Check sheet for the modelled part. Datum: model origin and axes. Units: mm. A direction names the side the tool comes from. Coordinates: 2 decimals unless noted, no trailing zeros. Loops run counter-clockwise (first coordinate to the right, second up) from the corner with the lowest first, then second, coordinate; pieces in that order, holes last.
from build123d import *

# Parameters (mm, degrees)
BOSS_EXTRUDE1_DEPTH = 10


# Read off the part's stored shape, not the designer's step: Imported1
with BuildPart() as part:
    # Sketch3 → Boss-Extrude1 (new body)
    with BuildSketch(Plane(origin=(14.999999665, 0, 0), x_dir=(0, 0, -1), z_dir=(1, 0, 0))):
        with BuildLine():
            Line((29.553098604, 349.581092596), (28.873996809, 356.511801481))
            ThreePointArc((28.873996809, 356.511801481), (26.617852211, 359.926750423), (22.636385635, 360.875427723))
            Line((22.636385635, 360.875427723), (-5.304185674, 354.369103909))
            Line((-5.304185674, 354.369103909), (-10.304185562, 354.369103909))
            Line((-10.304185562, 354.369103909), (-10.304185562, 214.764729142))
            Line((-10.304185562, 214.764729142), (43.492022902, 215.872973204))
            ThreePointArc((43.492022902, 215.872973204), (47.063645136, 218.78911025), (48.163164407, 223.266988993))
            Line((48.163164407, 223.266988993), (46.73166573, 228.318288922))
            Line((46.73166573, 228.318288922), (44.741906226, 228.116184473))
            Line((44.741906226, 228.116184473), (45.146130025, 224.136650562))
            Line((45.146130025, 224.136650562), (43.445847929, 219.970226288))
            Line((43.445847929, 219.970226288), (38.855373859, 219.58476305))
            Line((38.855373859, 219.58476305), (38.622945547, 221.872985363))
            Line((38.622945547, 221.872985363), (5.372944754, 221.872985363))
            Line((5.372944754, 221.872985363), (5.372944288, 349.872976542))
            Line((5.372944288, 349.872976542), (20.103313029, 353.819966316))
            Line((20.103313029, 353.819966316), (19.735585898, 356.090396643))
            Line((19.735585898, 356.090396643), (24.27472733, 356.836169958))
            Line((24.27472733, 356.836169958), (26.93930082, 353.209882975))
            Line((26.93930082, 353.209882975), (27.578826994, 349.261313677))
            Line((27.578826994, 349.261313677), (29.553098604, 349.581092596))
        make_face()
        Polygon((-5.304185562, 221.872985363), (0.372943822, 221.872985363), (0.372943822, 348.53323067), (-5.304185562, 347.01204868), align=None, mode=Mode.SUBTRACT)
    extrude(amount=BOSS_EXTRUDE1_DEPTH)


solid = part.part
(1) Section check D-D, the plane y = 226. Enter the section's corners in (x, z), plus the area to 3 significant figures.
(2) Scan lines: line 1 along Z through (x, y) = (24, 237); line 2 along Y through (x, z) = (19.75, -26.5); line 3 along Y through (x, z) = (20.5, -10.5). Record each from-to range of solid material in increasing order.
(3) Gauge pin test, flat ends, axial feed: P1, Ø3, axis at x = 20.5, z = 2, coming from the +Y side; P2, Ø5, axis at x = 22, y = 299, coming from the -Z side; P3, Ø5.5, axis at x = 19.5, z = 9, coming from the +Y side. Record the tip position at first contact, or that the pin passes through.
(4) Set-up check for faces 5 (the face through (20, 221.873, 3)), 6 (the face through (15, 283, -4)), 7 (the face through (20, 354.369, 8)): record each of +Z, -Z, +X, -X, +Y, -Y from which the full face is reachable in a straight line by a thin tool's end or side.
(5) Draft check along Y on faces 1 (the face through (19.93, 219.78, -41.18)), 2 (the face through (19.93, 355.048, -25.588)), 3 (the face through (19.93, 351.82, -12.64)), 4 (the face through (25, 283, -4)). Enter one of: pulls with the +Y half, pulls with the -Y half, needs draft (parallel to the pull), parting line crosses it, or undercut.
(6) Section check C-C, the plane z = -11.5. Enter the section's corners in (x, y), plus the area to 3 significant figures.
(7) Section check B-B, the plane x = 16.75. Enter the section's corners in (y, z), plus the area to 3 significant figures.
(8) Section check A-A, the plane y = 328. Enter the section's corners in (x, z).
Determined:
1. outline: (15, -47.39) - (25, -47.39) - (25, -44.96) - (15, -44.96) - close; (15, -5.37) - (25, -5.37) - (25, -0.37) - (15, -0.37) - close; (15, 5.3) - (25, 5.3) - (25, 10.3) - (15, 10.3) - close
1. area: 124 mm2
2. line 1: z = -5.37 to -0.37, 5.3 to 10.3
2. line 2: y = 215.52 to 221.87, 353.81 to 360.01
2. line 3: y = 215.19 to 221.87, 351.25 to 358.05
3. P1: stops at y = 355.49
3. P2: stops at z = -5.37
3. P3: stops at y = 354.37
4. face 5: +X, -X
4. face 6: +Z, -Z, -X, +Y, -Y
4. face 7: +Z, +X, -X, +Y
5. face 1: pulls with the +Y half
5. face 2: undercut
5. face 3: undercut
5. face 4: needs draft
6. outline: (15, 215.21) - (25, 215.21) - (25, 221.87) - (15, 221.87) - close; (15, 351.51) - (25, 351.51) - (25, 358.28) - (15, 358.28) - close
6. area: 134 mm2
7. outline: (214.76, 10.3) - (215.87, -43.49) arc R7.27 ccw to (223.27, -48.16) - (228.32, -46.73) - (228.12, -44.74) - (224.14, -45.15) - (219.97, -43.45) - (219.58, -38.86) - (221.87, -38.62) - (221.87, -5.37) - (349.87, -5.37) - (353.82, -20.1) - (356.09, -19.74) - (356.84, -24.27) - (353.21, -26.94) - (349.26, -27.58) - (349.58, -29.55) - (356.51, -28.87) arc R5.57 ccw to (360.88, -22.64) - (354.37, 5.3) - (354.37, 10.3) - close; hole (221.87, -0.37) - (348.53, -0.37) - (347.01, 5.3) - (221.87, 5.3) - close
7. area: 1,900 mm2
8. outline: (15, -5.37) - (25, -5.37) - (25, -0.37) - (15, -0.37) - close; (15, 5.3) - (25, 5.3) - (25, 10.3) - (15, 10.3) - close
